from build123d import *

# Parameters (mm, degrees)
ESQUISSE1_W                                         = 120
ESQUISSE1_H                                         = 50
BOSS_EXTRU_1_DEPTH                                  = 10
ESQUISSE2_W                                         = 25
ESQUISSE2_H                                         = 30
ENL_V_MAT_EXTRU_1_DEPTH                             = 10
CSK_FOR_M5_COUNTERSUNK_FLAT_HEAD_SCREW1_D           = 5.5
CSK_FOR_M5_COUNTERSUNK_FLAT_HEAD_SCREW1_CSINK_D     = 10.4
CSK_FOR_M5_COUNTERSUNK_FLAT_HEAD_SCREW1_CSINK_ANGLE = 90


with BuildPart() as part:
    # Esquisse1 → Boss.-Extru.1 (new body)
    with BuildSketch(Plane.XY):
        Rectangle(ESQUISSE1_W, ESQUISSE1_H)
    extrude(amount=BOSS_EXTRU_1_DEPTH)

    # Esquisse2 → Enlèv. mat.-Extru.1 (cut)
    with BuildSketch(Plane.XY.offset(10)):
        with Locations((-35.5, 0)):
            Rectangle(ESQUISSE2_W, ESQUISSE2_H)
    extrude(amount=-ENL_V_MAT_EXTRU_1_DEPTH, mode=Mode.SUBTRACT)

    # CSK for M5 Countersunk Flat Head Screw1 (through all)
    with Locations(Plane.XY.offset(10)):
        with Locations((16, 0), (40, 0)):
            CounterSinkHole(CSK_FOR_M5_COUNTERSUNK_FLAT_HEAD_SCREW1_D / 2, CSK_FOR_M5_COUNTERSUNK_FLAT_HEAD_SCREW1_CSINK_D / 2, counter_sink_angle=CSK_FOR_M5_COUNTERSUNK_FLAT_HEAD_SCREW1_CSINK_ANGLE)


solid = part.part
For this review, take the finished solid that the model builds, in its own axes (mm). A direction names the side the tool comes from. Give positions to 0.01 mm unless a question says otherwise; leave off trailing zeros. Loops run counter-clockwise (first coordinate to the right, second up) from the corner with the lowest first, then second, coordinate; pieces in that order, holes last.
Item 1: Insertion check: pin 1 (7 mm diameter, centred on x = 40, y = 0, fed in from -Z); pin 2 (7 mm diameter, centred on x = 16, y = 0, fed in from +Z). Each pin has a flat end and moves straight along its axis. Give the tip position at first contact, or say it passes through.
Item 2: Tool access review of faces 1 (the flat face through (-23, 0, 5)), 2 (the conical face through (42.9, 0.1, 7.7)): name each direction out of +Z, -Z, +X, -X, +Y, -Y from which nothing blocks a thin tool from reaching the whole face with its end or side.
Item 3: For line 1 along X through (y, z) = (0, 4.25); line 2 along X through (y, z) = (10, 7); line 3 along Y through (x, z) = (-42.5, 6.5), list the stretches that pass through material, from the lowest coordinate up.
Item 4: Take a section at D-D, the plane y = -13. State the section outline as (x, z) points, and give its area (3 significant figures).
Item 5: Draft analysis for pull direction Y (two halves, no side actions). For faces 3 (the flat face through (-1, -25, 5)), 4 (the conical face through (13.35, -1.1, 7.67)), 5 (the flat face through (60, 0, 5)), state which applies: +Y half, -Y half, draft (parallel to the pull), parting line (faces both ways), or undercut.
Item 6: Take a section at C-C, the plane x = -44. State the section outline as (y, z) points, and give its area (3 significant figures).
Item 7: Take a section at B-B, the plane z = 8.75. State the section outline as (x, y) points, and give its area (3 significant figures).
Item 8: Take a section at A-A, the plane y = 0. State the section outline as (x, z) points, and give its area (3 significant figures).
Calculated:
1. pin 1: stops at z = 0
1. pin 2: stops at z = 8.3
2. face 1: +Z, -Z
2. face 2: +Z
3. line 1: x = -60 to -48, -23 to 13.25, 18.75 to 37.25, 42.75 to 60
3. line 2: x = -60 to -48, -23 to 60
3. line 3: y = -25 to -15, 15 to 25
4. outline: (-60, 0) - (-48, 0) - (-48, 10) - (-60, 10) - close; (-23, 0) - (60, 0) - (60, 10) - (-23, 10) - close
4. area: 950 mm2
5. face 3: -Y half
5. face 4: undercut
5. face 5: draft
6. outline: (-25, 0) - (-15, 0) - (-15, 10) - (-25, 10) - close; (15, 0) - (25, 0) - (25, 10) - (15, 10) - close
6. area: 200 mm2
7. outline: (-60, -25) - (60, -25) - (60, 25) - (-60, 25) - close; hole (-48, -15) - (-23, -15) - (-23, 15) - (-48, 15) - close; hole circle Ø7.9 at (16, 0); hole circle Ø7.9 at (40, 0)
7. area: 5,150 mm2
8. outline: (-60, 0) - (-48, 0) - (-48, 10) - (-60, 10) - close; (-23, 0) - (13.25, 0) - (13.25, 7.55) - (10.8, 10) - (-23, 10) - close; (18.75, 0) - (37.25, 0) - (37.25, 7.55) - (34.8, 10) - (21.2, 10) - (18.75, 7.55) - close; (42.75, 0) - (60, 0) - (60, 10) - (45.2, 10) - (42.75, 7.55) - close
8. area: 828 mm2
